Here's how the part is built. I have some questions about the finished solid (model axes, mm). A direction names the side the tool comes from. Coordinates: 2 decimals unless noted, no trailing zeros. Write each loop counter-clockwise with the first axis right and the second up, starting at its lowest first coordinate (ties: lowest second). Pieces come first, ordered by that corner, then holes. Notation, with made-up numbers: (-22, -39.75) -> (26, -39.75) arc R29 ccw to (26, -15.75) -> close; hole circle Ø11 at (18.5, 81). An arc over 180 degrees is marked (long way). Use a Markdown table: item, result. Add a question column.
Item 1: Imagine slicing it at C-C, the plane z = -6.5. Write out the boundary of the cut face in (x, y).
Item 2: On a 3-axis mill with a long thin cutter (end or side, diameter ignored), from which of +Z, -Z, +X, -X, +Y, -Y can I reach the whole of each face in a straight line? I mean faces 4 (the flat face through (-1.293, 0.76, 3.521)), 5 (the flat face through (0, -2, 5)), 6 (the flat face through (0, -2, 0)). Say none if no direction works.
Item 3: Imagine slicing it at A-A, the plane x = 0. Write out the boundary of the cut face in (y, z).
Item 4: If we mould it in two halves opening along X, with no side actions, what happens to faces 1 (the cylindrical face through (-0.54, -2.44, 2.46)), 2 (the flat face through (0, 0, -15)), 3 (the flat face through (0, 1.5, 4))? For each: pulls with the +X half, pulls with the -X half, needs draft (parallel to the pull), parting line crosses it, or undercut.
Item 5: Will these pins go through, and if not, where does the flat tip stop? pin 1 Ø1 at (x, z) = (1.5, -4.5) entering from +Y; pin 2 Ø1 at (y, z) = (-1, 0) entering from -X; pin 3 Ø1 at (x, y) = (0.5, -0.5) entering from +Z.
Item 6: Imagine slicing it at D-D, the plane x = 2.15. Write out the boundary of the cut face in (y, z).
Item 7: If I drill on line 1 along Z through (x, y) = (-0.3, 1.05); line 2 along Y through (x, z) = (-1.8, 3); line 3 along Y through (x, z) = (-0.1, -4.5), over which ranges is the centre line in solid material (lowest first)? Write a range as from..to.
Item 8: Imagine slicing it at B-B, the plane y = -1.2. Write out the boundary of the cut face in (x, z).
```python
from build123d import *

# Parameters (mm, degrees)
F0_R     = 1.5
F1_DEPTH = 15
F2_R     = 2.5
F2_R_2   = 1.5
F3_DEPTH = 5
F5_DEPTH = 3


with BuildPart() as f1:
    # F0 (on Top) → F1 (new body)
    with BuildSketch(Plane.XY):
        Circle(F0_R)
    extrude(amount=-F1_DEPTH)

    # F2 (on face) → F3 (join)
    with BuildSketch(Plane.XY):
        Circle(F2_R)
        Circle(F2_R_2, mode=Mode.SUBTRACT)
        Circle(F2_R_2)
    extrude(amount=F3_DEPTH)

    # F4 (on face) → F5 (cut)
    with BuildSketch(Plane.XY.offset(5)):
        Polygon((-0.866025, 1.5), (-1.732051, 0), (-0.866025, -1.5), (0.866025, -1.5), (1.732051, 0), (0.866025, 1.5), align=None)
    extrude(amount=-F5_DEPTH, mode=Mode.SUBTRACT)


solid = f1.part
```
Ans:
| question | item | result |
|---|---|---|
| 1 | outline | circle Ø3 at (0, 0) |
| 2 | face 4 | +Z |
| 2 | face 5 | +Z, +X, -X, +Y, -Y |
| 2 | face 6 | -Z |
| 3 | outline | (-2.5, 0) -> (-1.5, 0) -> (-1.5, -15) -> (1.5, -15) -> (1.5, 0) -> (2.5, 0) -> (2.5, 5) -> (1.5, 5) -> (1.5, 2) -> (-1.5, 2) -> (-1.5, 5) -> (-2.5, 5) -> close |
| 4 | face 1 | parting line crosses it |
| 4 | face 2 | needs draft |
| 4 | face 3 | undercut |
| 5 | pin 1 | stops at y = 1.12 |
| 5 | pin 2 | stops at x = -2.45 |
| 5 | pin 3 | stops at z = 2 |
| 6 | outline | (-1.28, 0) -> (1.28, 0) -> (1.28, 5) -> (-1.28, 5) -> close |
| 7 | line 1 | z = -15..2 |
| 7 | line 2 | y = -1.73..1.73 |
| 7 | line 3 | y = -1.5..1.5 |
| 8 | outline | (-2.19, 0) -> (-0.9, 0) -> (-0.9, -15) -> (0.9, -15) -> (0.9, 0) -> (2.19, 0) -> (2.19, 5) -> (1.04, 5) -> (1.04, 2) -> (-1.04, 2) -> (-1.04, 5) -> (-2.19, 5) -> close |
